Source: CAD feature listing. Evaluate the final solid. Frame: model axes, mm. A direction names the side the tool comes from. Give positions to 0.01 mm unless a question says otherwise; leave off trailing zeros. Loops run counter-clockwise (first coordinate to the right, second up) from the corner with the lowest first, then second, coordinate; pieces in that order, holes last. Notation, with made-up numbers: (45.5, 84) -> (102.5, 84) arc R16 cw to (102.5, 91) -> close; hole circle Ø11 at (69.5, -4). An arc over 180 degrees is marked (long way). Put each result on its own line as item: value.
```python
from build123d import *

# Parameters (mm, degrees)
BOSS_EXTRUDE1_DEPTH = 203.2
FILLET1_R           = 2.54
SKETCH2_R           = 2.667
CUT_EXTRUDE1_DEPTH  = 11.43


with BuildPart() as part:
    # Sketch1 → Boss-Extrude1 (new body)
    with BuildSketch(Plane.XY):
        with BuildLine():
            Line((-12.7, 73.846320157), (12.7, 73.846320157))
            Line((12.7, 73.846320157), (15.605843118, 90.742841512))
            ThreePointArc((15.605843118, 90.742841512), (23.776020133, 88.952270863), (31.75, 86.427675689))
            Line((31.75, 86.427675689), (31.75, 99.102275689))
            Line((31.75, 99.102275689), (-31.75, 99.102275689))
            Line((-31.75, 99.102275689), (-31.75, 86.427675689))
            ThreePointArc((-31.75, 86.427675689), (-23.776020133, 88.952270863), (-15.605843118, 90.742841512))
            Line((-15.605843118, 90.742841512), (-12.7, 73.846320157))
        make_face()
    extrude(amount=BOSS_EXTRUDE1_DEPTH)

    # Fillet1
    fillet1_edges = [part.edges().sort_by_distance(p)[0] for p in [
        (12.7, 73.846320157, 101.6),
        (-12.7, 73.846320157, 101.6),
        (-15.605843118, 90.742841512, 101.6),
        (15.605843118, 90.742841512, 101.6),
    ]]
    fillet(fillet1_edges, radius=FILLET1_R)

    # Sketch2 → Cut-Extrude1 (cut)
    with BuildSketch(Plane.XY.offset(203.2)):
        with Locations((-8.89, 92.752275689)):
            Circle(SKETCH2_R)
        with Locations((8.89, 92.752275689)):
            Circle(SKETCH2_R)
        with Locations((0, 80.052275689)):
            Circle(SKETCH2_R)
    extrude(amount=-CUT_EXTRUDE1_DEPTH, mode=Mode.SUBTRACT)


solid = part.part
```
(1) Section B-B on x = -23. Return loops of the section in (y, z).
Calculated:
outline: (89.16, 0) -> (99.1, 0) -> (99.1, 203.2) -> (89.16, 203.2) -> close
(2) Section C-C on x = 26. Return loops of the section in (y, z), then the cut area to 3 significant figures.
Calculated:
outline: (88.33, 0) -> (99.1, 0) -> (99.1, 203.2) -> (88.33, 203.2) -> close
area: 2,190 mm²
(3) Line query: probe 1 along Y at (x, z) = (-8.89, 195.5); probe 2 along Z at (x, y) = (1, 80.5); probe 3 along Y at (x, z) = (26.5, 73). Output: solid intervals per line, ascending. Write a range as from..to.
Calculated:
probe 1: y = 73.85..90.09, 95.42..99.1
probe 2: z = 0..191.77
probe 3: y = 88.18..99.1
(4) First-contact query: P1, Ø5, axis at x = -14, z = 165.5, coming from the -Y side; P2, Ø2.5, axis at x = 0.5, y = 79, coming from the +Z side; P3, Ø1.5, axis at y = 82.5, z = 118.5, coming from the +X side. Flat tips, straight axial feed; report the tip coordinate or a pass-through.
Calculated:
P1: stops at y = 74.03
P2: stops at z = 191.77
P3: stops at x = 14.32
(5) Draft query along X for faces 1 (the flat face through (-31.75, 93, 100)), 2 (the cylindrical face through (-0.347, 82.697, 197.565)), 3 (the flat face through (31.75, 93, 100)), 4 (the flat face through (0, 99.102, 100)). Return one class per face: released by +X, released by -X, zero draft, split by the parting line, or undercut.
Calculated:
face 1: released by -X
face 2: undercut
face 3: released by +X
face 4: zero draft
(6) Reachability of faces 5 (the flat face through (0, 89, 0)), 6 (the cylindrical face through (-25.13, 88.58, 100.18)), 7 (the flat face through (9, 93, 191.77)) from +Z, -Z, +X, -X, +Y, -Y: full face, straight path, thin tool, end or side. Return the list, or none.
Calculated:
face 5: -Z, +X, -X, +Y, -Y
face 6: +Z, -Z, -Y
face 7: +Z
(7) Section A-A on z = 112. Return loops of the section in (x, y) (3 decimals).
Calculated:
outline: (-31.75, 86.428) arc R92.075 cw to (-18.174, 90.264) arc R2.54 cw to (-15.169, 88.204) -> (-13.063, 75.956) arc R2.54 ccw to (-10.56, 73.846) -> (10.56, 73.846) arc R2.54 ccw to (13.063, 75.956) -> (15.169, 88.204) arc R2.54 cw to (18.174, 90.264) arc R92.075 cw to (31.75, 86.428) -> (31.75, 99.102) -> (-31.75, 99.102) -> close
